from build123d import *

# Parameters (mm, degrees)
F1_DEPTH = 25.4
F2_R     = 12.69999
F3_R     = 3.175
F4_DEPTH = 6.351


# Not quite as in the source:
# - a fillet or chamfer is up to 0.001 mm smaller than in the source, because OpenCascade refuses the exact size


with BuildPart() as f1:
    # F0 (on Front) → F1 (new body)
    with BuildSketch(Plane.XZ):
        Polygon((31.75, 0), (0, 0), (0, -6.35), (38.1, -6.35), (38.1, 19.05), (63.5, 19.05), (63.5, -6.35), (101.6, -6.35), (101.6, 0), (69.85, 0), (69.85, 25.4), (31.75, 25.4), align=None)
    extrude(amount=F1_DEPTH)

    # F2 (radius 12.7 in the source; OpenCascade refuses exactly that, so slightly less here)
    f2_edges = [f1.edges().sort_by_distance(p)[0] for p in [
        (31.75, -12.7, 25.4),
        (38.1, -12.7, 19.05),
        (69.85, -12.7, 25.4),
        (63.5, -12.7, 19.05),
        (63.5, -12.7, -6.35),
        (69.85, -12.7, 0),
        (38.1, -12.7, -6.35),
        (31.75, -12.7, 0),
    ]]
    fillet(f2_edges, radius=F2_R)

    # F3 (on face) → F4 (cut, through all)
    with BuildSketch(Plane.XY):
        with Locations((9.525, -12.7)):
            Circle(F3_R)
        with Locations((92.075, -12.7)):
            Circle(F3_R)
    extrude(amount=-F4_DEPTH, mode=Mode.SUBTRACT)


solid = f1.part
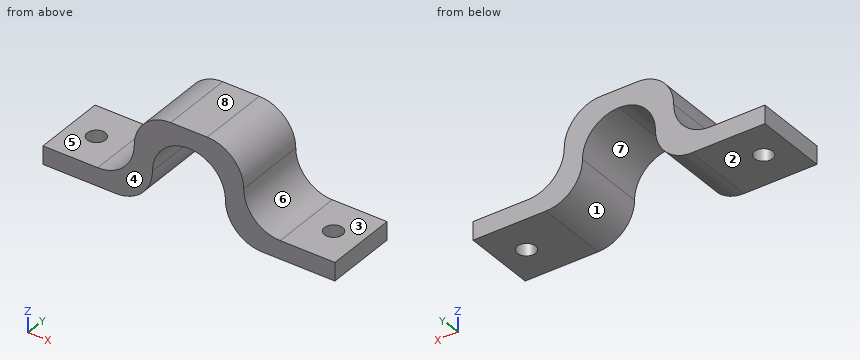
Geometry: final body of the model. Coordinates: model frame, mm. Face numbers are marked on the shaded views. A direction names the side the tool comes from. Give positions to 0.01 mm unless a question says otherwise; leave off trailing zeros. Write each loop counter-clockwise with the first axis right and the second up, starting at its lowest first coordinate (ties: lowest second). Pieces come first, ordered by that corner, then holes. Notation, with made-up numbers: (76, -26) -> (83, -26) arc R23 cw to (83, -1) -> close; hole circle Ø5 at (-18, -33.75). An arc over 180 degrees is marked (long way). Answer as a JSON object with one key per item and string values.
1. Cut plane A-A on y = -12.7. Count the separate pieces of the cut face and the enclosed holes in it, and give its area (3 significant figures).
Ans:
{"separate pieces": "3", "enclosed holes": "0", "area": "887 mm^2"}
2. Mould query, pull axis X, two halves, no side actions, for the marked faces 6, 7 and 8. Classes: pulls with the +X half, pulls with the -X half, needs draft (parallel to the pull), parting line crosses it, or undercut.
Ans:
{"face 6": "pulls with the +X half", "face 7": "undercut", "face 8": "needs draft"}
3. Cut plane C-C on x = 91.5. Output: boundary loops of the cut face in (y, z).
Ans:
{"outline": "(-25.4, -6.35) -> (-15.82, -6.35) -> (-15.82, 0) -> (-25.4, 0) -> close; (-9.58, -6.35) -> (0, -6.35) -> (0, 0) -> (-9.58, 0) -> close"}
4. Cut plane B-B on z = 7.5. Output: boundary loops of the cut face in (x, y).
Ans:
{"outline": "(30.64, -25.4) -> (38.15, -25.4) -> (38.15, 0) -> (30.64, 0) -> close; (63.45, -25.4) -> (70.96, -25.4) -> (70.96, 0) -> (63.45, 0) -> close"}
5. Access query for the marked faces 1, 2, 3, 4 and 5. Directions: +Z, -Z, +X, -X, +Y, -Y. A direction counts if a zero-diameter tool reaches every point of the face in a straight line with its end or side. Return the directions, or none.
Ans:
{"face 1": "-Z, +Y, -Y", "face 2": "-Z, +X, -X, +Y, -Y", "face 3": "+Z, +X, +Y, -Y", "face 4": "+Z, -Z, +X, -X, -Y", "face 5": "+Z, -X, +Y, -Y"}
6. Contact query for flat-ended pins moving along their axis: pin 1 (2 mm diameter, centred on y = -5.5, z = 7, fed in from +X); pin 2 (5 mm diameter, centred on x = 92.075, y = -12.7, fed in from -Z); pin 3 (3 mm diameter, centred on x = 19, y = -15, fed in from +Z); pin 4 (7.5 mm diameter, centred on x = 9.525, y = -12.7, fed in from -Z). Output: stop coordinate, or through.
Ans:
{"pin 1": "stops at x = 71.76", "pin 2": "passes through", "pin 3": "stops at z = 0.08", "pin 4": "stops at z = -6.35"}
7. Ray query, probe 1 along X at (y, z) = (-11.75, -2.5); probe 2 along X at (y, z) = (-14, 1.5); probe 3 along Z at (x, y) = (95, -18.75). Return the intervals inside material, ascending. Write a range as from..to.
Ans:
{"probe 1": "x = 0..6.5, 12.55..34.51, 67.09..89.05, 95.1..101.6", "probe 2": "x = 25.04..37.14, 64.46..76.56", "probe 3": "z = -6.35..0"}
